from build123d import *

# Parameters (mm, degrees)
SKETCH1_W             = 14
SKETCH1_H             = 20
BOSS_EXTRUDE1_DEPTH   = 6.35
SKETCH2_W             = 2.55
SKETCH2_H             = 1.754165379
BOSS_EXTRUDE2_DEPTH   = 2
SKETCH3_W             = 2.55
SKETCH3_H             = 0.5
BOSS_EXTRUDE3_DEPTH   = 3
SKETCH4_W             = 0.5
SKETCH4_H             = 2.55
BOSS_EXTRUDE4_DEPTH   = 55
SKETCH5_W             = 3
SKETCH5_H             = 1
BOSS_EXTRUDE5_DEPTH   = 3
F_3_0MM_DOWEL_HOLE1_D = 3.5


with BuildPart() as part:
    # Sketch1 → Boss-Extrude1 (new body)
    with BuildSketch(Plane.XY):
        with Locations((7, 10)):
            Rectangle(SKETCH1_W, SKETCH1_H)
    extrude(amount=-BOSS_EXTRUDE1_DEPTH)

    # Sketch2 → Boss-Extrude2 (add)
    with BuildSketch(Plane.ZY):
        with Locations((-3.175, 7.877082689)):
            Rectangle(SKETCH2_W, SKETCH2_H)
    extrude(amount=BOSS_EXTRUDE2_DEPTH)

    # Sketch3 → Boss-Extrude3 (add)
    with BuildSketch(Plane.ZY):
        with Locations((-3.175, 4.25)):
            Rectangle(SKETCH3_W, SKETCH3_H)
    extrude(amount=BOSS_EXTRUDE3_DEPTH)

    # Sketch4 → Boss-Extrude4 (add)
    with BuildSketch(Plane(origin=(0, 4.5, 0), x_dir=(1, 0, 0), z_dir=(0, 1, 0))):
        with Locations((-2.75, 3.175)):
            Rectangle(SKETCH4_W, SKETCH4_H)
    extrude(amount=BOSS_EXTRUDE4_DEPTH)

    # Sketch5 → Boss-Extrude5 (add)
    with BuildSketch(Plane(origin=(14, 0, 0), x_dir=(0, 0, -1), z_dir=(1, 0, 0))):
        with Locations((3.175, 3.5)):
            Rectangle(SKETCH5_W, SKETCH5_H)
        with Locations((3.175, 10)):
            Rectangle(SKETCH5_W, SKETCH5_H)
        with Locations((3.175, 16.5)):
            Rectangle(SKETCH5_W, SKETCH5_H)
    extrude(amount=BOSS_EXTRUDE5_DEPTH)

    # Ø3.0mm Dowel Hole1 (through all)
    with Locations(Plane(origin=(10.5, 15, 0), x_dir=(1, 0, 0), z_dir=(0, 0, 1))):
        with Locations((0, 0), (0, -10)):
            Hole(F_3_0MM_DOWEL_HOLE1_D / 2)


solid = part.part
Can you work these out from the model? Positions are in its coordinate system, mm. A direction names the side the tool comes from. Coordinates: 2 decimals unless noted, no trailing zeros. Write each loop counter-clockwise with the first axis right and the second up, starting at its lowest first coordinate (ties: lowest second). Pieces come first, ordered by that corner, then holes. Notation, with made-up numbers: (-35, 19.25) -> (3, 19.25) arc R13 cw to (3, 31.25) -> close; hole circle Ø7 at (47.5, 16). An arc over 180 degrees is marked (long way). Write each question's results on one line, items separated by ' | '. Start each with the question number.
Item 1: If we section it at B-B, the plane y = 8: Write out the boundary of the cut face in (x, z), and give its area (3 significant figures).
Item 2: Please list where these lines run through material, in increasing order: probe 1 along Y at (x, z) = (10.5, -4.5); probe 2 along Y at (x, z) = (15.75, -4); probe 3 along Y at (x, z) = (8.5, -1.5).
Item 3: If we section it at D-D, the plane z = -0.75: Write out the boundary of the cut face in (x, y), and give its area (3 significant figures).
Item 4: On a 3-axis mill with a long thin cutter (end or side, diameter ignored), from which of +Z, -Z, +X, -X, +Y, -Y can I reach the whole of each face in a straight line? I mean faces 1 (the flat face through (-1, 8, -1.9)), 2 (the flat face through (15, 3, -3)), 3 (the flat face through (-1, 8, -4.45)), 4 (the flat face through (15, 10.5, -3)). Say none if no direction works.
Item 5: If we section it at C-C, the plane y = 15: Write out the boundary of the cut face in (x, z).
Item 6: If we section it at A-A, the plane x = 15: Write out the boundary of the cut face in (y, z) (3 decimals).
Item 7: Thinking about a two-plate mould opening in X: for faces 5 (the flat face through (-2, 8, -3)), 6 (the flat face through (7, 10, 0)), 7 (the flat face through (-3, 31, -3)), which applies, released by +X, released by -X, zero draft, split by the parting line, or undercut?
Item 8: I'm going to push flat-ended pins straight in: P1, Ø2.5, axis at x = -1.5, y = 26, coming from the -Z side; P2, Ø1.1, axis at x = 15.5, y = 16.5, coming from the +Z side (3 decimals); P3, Ø2.5, axis at x = 15, z = -2.5, coming from the +Y side. Where does each tip first touch, or does it pass through?
Answer block:
1) outline: (-3, -4.45) -> (-2.5, -4.45) -> (-2.5, -1.9) -> (-3, -1.9) -> close; (-2, -4.45) -> (0, -4.45) -> (0, -6.35) -> (14, -6.35) -> (14, 0) -> (0, 0) -> (0, -1.9) -> (-2, -1.9) -> close | area: 95.3 mm²
2) probe 1: 0 to 3.25, 6.75 to 13.25, 16.75 to 20 | probe 2: 3 to 4, 9.5 to 10.5, 16 to 17 | probe 3: 0 to 20
3) outline: (0, 0) -> (14, 0) -> (14, 20) -> (0, 20) -> close; hole circle Ø3.5 at (10.5, 5); hole circle Ø3.5 at (10.5, 15) | area: 261 mm²
4) face 1: +Z, -X, +Y, -Y | face 2: +Z, -Z, +X, -Y | face 3: -Z, -X, +Y, -Y | face 4: +Z, -Z, +X
5) outline: (-3, -4.45) -> (-2.5, -4.45) -> (-2.5, -1.9) -> (-3, -1.9) -> close; (0, -6.35) -> (8.75, -6.35) -> (8.75, 0) -> (0, 0) -> close; (12.25, -6.35) -> (14, -6.35) -> (14, 0) -> (12.25, 0) -> close
6) outline: (3, -4.675) -> (4, -4.675) -> (4, -1.675) -> (3, -1.675) -> close; (9.5, -4.675) -> (10.5, -4.675) -> (10.5, -1.675) -> (9.5, -1.675) -> close; (16, -4.675) -> (17, -4.675) -> (17, -1.675) -> (16, -1.675) -> close
7) face 5: undercut | face 6: zero draft | face 7: released by -X
8) P1: z = -4.45 | P2: z = -1.675 | P3: y = 20
